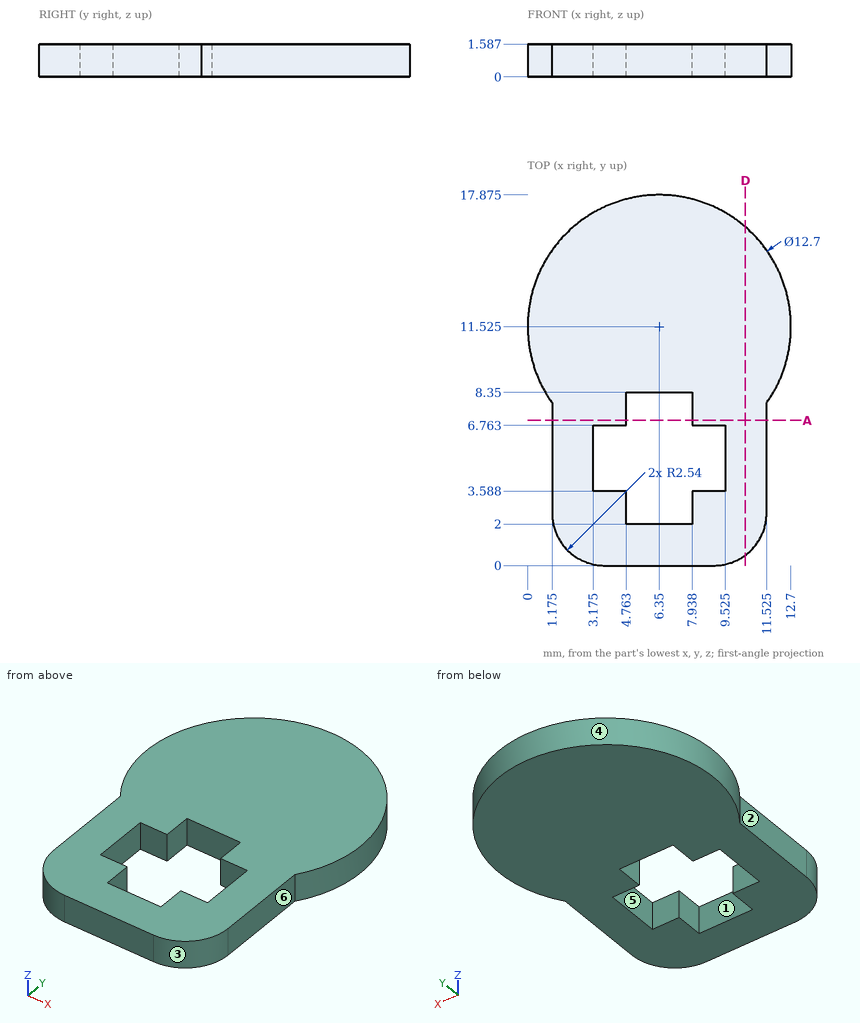
Study the drawing (mm; zero at the part's minimum x, y, z) and answer. A direction names the side the tool comes from. Give positions to 0.01 mm unless a question says otherwise; leave off trailing zeros. Loops run counter-clockwise (first coordinate to the right, second up) from the corner with the lowest first, then second, coordinate; pieces in that order, holes last. Notation, with made-up numbers: (23.5, 85.25) - (28.5, 85.25) arc R12 ccw to (28.5, 97.25) - close; hole circle Ø6 at (-22.75, 59.5). An arc over 180 degrees is marked (long way). Return JSON: item names as keys, results as strings. Group by question number.
1. Which of the six approach directions +Z, -Z, +X, -X, +Y, -Y give full straight-line access (tool end or side, diameter ignored) to the marked faces 1, 2 and 3?
2. Given pin 1 Ø0.8 at (x, z) = (8.5, 1) entering from +Y; pin 2 Ø0.8 at (y, z) = (4.5, 1) entering from -X (1 decimal); pin 3 Ø0.5 at (x, z) = (4.5, 0.5) entering from +Y, each flat-ended and moving along its own axis, determine where each tip first touches the part or whether it passes through.
3. Find section A-A (y = 7). Write down the section's boundary in (x, z) (1 decimal), then the cut area to 3 significant figures.
4. Find section D-D (x = 10.5). Write down the section's boundary in (y, z).
5. Straight lines are drawn through the part: line 1 (X direction, y = 3.5, z = 1) (1 decimal); line 2 (X direction, y = 5.75, z = 0.7) (1 decimal); line 3 (Y direction, x = 7, z = 1.2). For each, find the intervals that lie inside material, in ascending order. Write a range as [from, to].
6. Determine the mould class of the marked faces 4, 5 and 6 for opening direction Y: pulls with the +Y half, pulls with the -Y half, needs draft (parallel to the pull), parting line crosses it, or undercut.
Verdict:
{
 "1": {"face 1": "+Z, -Z", "face 2": "+Z, -Z, -X, -Y", "face 3": "+Z, -Z, +X, -Y"},
 "2": {"pin 1": "stops at y = 17.63", "pin 2": "stops at x = 1.2", "pin 3": "stops at y = 17.67"},
 "3": {"outline": "(1.2, 0) - (4.8, 0) - (4.8, 1.6) - (1.2, 1.6) - close; (7.9, 0) - (11.5, 0) - (11.5, 1.6) - (7.9, 1.6) - close", "area": "11.4 mm^2"},
 "4": {"outline": "(0.5, 0) - (16.33, 0) - (16.33, 1.59) - (0.5, 1.59) - close"},
 "5": {"line 1": "x = [1.2, 4.8], [7.9, 11.5]", "line 2": "x = [1.2, 3.2], [9.5, 11.5]", "line 3": "y = [0, 2], [8.35, 17.84]"},
 "6": {"face 4": "parting line crosses it", "face 5": "undercut", "face 6": "needs draft"}
}
